from build123d import *

# Parameters (mm, degrees)
F0_W     = 906.4625
F0_H     = 547.6875
F1_DEPTH = 244.475
F2_W     = 21.43125
F2_H     = 490.5375
F3_DEPTH = 244.476
F4_R     = 25.4
F5_W     = 793.75
F5_H     = 455.6125
F6_DEPTH = 228.6
F7_R     = 25.4


with BuildPart() as f1:
    # F0 (on Top) → F1 (new body)
    with BuildSketch(Plane.XY):
        with Locations((15.469722, -72.404954)):
            Rectangle(F0_W, F0_H)
    extrude(amount=F1_DEPTH)

    # F2 (on face) → F3 (cut, through all)
    with BuildSketch(Plane.XY.offset(244.475)):
        with Locations((-427.045903, -43.829954)):
            Rectangle(F2_W, F2_H)
        with Locations((457.985347, -43.829954)):
            Rectangle(F2_W, F2_H)
    extrude(amount=-F3_DEPTH, mode=Mode.SUBTRACT)

    # F4
    f4_edges = [f1.edges().sort_by_distance(p)[0] for p in [
        (-437.761528, -346.248704, 122.2375),
        (468.700972, -346.248704, 122.2375),
    ]]
    fillet(f4_edges, radius=F4_R)

    # F5 (on face) → F6 (cut)
    with BuildSketch(Plane.XY.offset(244.475)):
        with Locations((15.469722, -61.292454)):
            Rectangle(F5_W, F5_H)
    extrude(amount=-F6_DEPTH, mode=Mode.SUBTRACT)

    # F7
    f7_edges = [f1.edges().sort_by_distance(p)[0] for p in [
        (412.344722, 166.513796, 130.175),
        (-381.405278, 166.513796, 130.175),
        (-381.405278, -289.098704, 130.175),
        (412.344722, -289.098704, 130.175),
    ]]
    fillet(f7_edges, radius=F7_R)


solid = f1.part
Here's how the part is built. I have some questions about the finished solid (model axes, mm). A direction names the side the tool comes from. Give positions to 0.01 mm unless a question says otherwise; leave off trailing zeros. Order: outer loops, then holes, each group sorted by start corner. A loop starts at its lowest first (then second) coordinate and runs counter-clockwise, first axis right, second up. Notation, with made-up numbers: (78.5, 7.25) -> (113.5, 7.25) arc R30 cw to (113.5, 36.25) -> close; hole circle Ø4 at (84.5, 35). An arc over 180 degrees is marked (long way). Use a Markdown table: item, result. Add a question column.
Item 1: For faces 1 (the face through (13, -294, 244.475)), 2 (the face through (-373.767, -281.856, 128.575)), 3 (the face through (447.27, -47, 124)), which set-ups out of +Z, -Z, +X, -X, +Y, -Y let a thin tool reach every point of the face, with its end or its side?
Item 2: Imagine slicing it at B-B on y = -94.5. Please give me the cut outline in (x, z) (3 decimals).
Item 3: Imagine slicing it at A-A on x = -345. Please give me the cut outline in (y, z) (3 decimals).
Item 4: Imagine slicing it at C-C on z = 28. Please give me the cut outline in (x, y), plus the area to 3 significant figures.
Item 5: I need wall thicknesses on line 1 (Y direction, x = -330, z = 144.5); line 2 (X direction, y = -234, z = 31); line 3 (Z direction, x = 212, y = -5.5) (3 decimals). Which ranges of each line are inside material? Lowest first, please.
Item 6: If we mould it in two halves opening along X, with no side actions, what happens to faces 4 (the face through (461.06, -339.01, 123.95)), 5 (the face through (-427, -289.099, 124)), 6 (the face through (405.1, 158.88, 128.57))? For each: pulls with the +X half, pulls with the -X half, needs draft (parallel to the pull), parting line crosses it, or undercut.
Item 7: Will these pins go through, and if not, where does the flat tip stop? pin 1 (6.5 mm diameter, centred on x = -425, z = 166.5, fed in from +Y); pin 2 (4 mm diameter, centred on y = 106.5, z = 75, fed in from +X); pin 3 (6 mm diameter, centred on x = 320.5, y = -58.5, fed in from +Z) (3 decimals).
Data:
| question | item | result |
|---|---|---|
| 1 | face 1 | +Z, +X, -X, +Y, -Y |
| 1 | face 2 | +Z |
| 1 | face 3 | +Z, -Z, +X, +Y |
| 2 | outline | (-416.33, 0) -> (447.27, 0) -> (447.27, 244.475) -> (412.345, 244.475) -> (412.345, 15.875) -> (-381.405, 15.875) -> (-381.405, 244.475) -> (-416.33, 244.475) -> close |
| 3 | outline | (-346.249, 0) -> (201.439, 0) -> (201.439, 244.475) -> (166.514, 244.475) -> (166.514, 15.875) -> (-289.099, 15.875) -> (-289.099, 244.475) -> (-346.249, 244.475) -> close |
| 4 | outline | (-437.76, -320.85) arc R25.4 ccw to (-412.36, -346.25) -> (443.3, -346.25) arc R25.4 ccw to (468.7, -320.85) -> (468.7, -289.1) -> (447.27, -289.1) -> (447.27, 201.44) -> (-416.33, 201.44) -> (-416.33, -289.1) -> (-437.76, -289.1) -> close; hole (-381.41, -263.7) arc R25.4 ccw to (-356.01, -289.1) -> (386.94, -289.1) arc R25.4 ccw to (412.34, -263.7) -> (412.34, 141.11) arc R25.4 ccw to (386.94, 166.51) -> (-356.01, 166.51) arc R25.4 ccw to (-381.41, 141.11) -> close |
| 4 | area | 114,000 mm² |
| 5 | line 1 | y = -346.25 to -289.1, 166.51 to 201.44 |
| 5 | line 2 | x = -416.33 to -381.41, 412.34 to 447.27 |
| 5 | line 3 | z = 0 to 15.875 |
| 6 | face 4 | pulls with the +X half |
| 6 | face 5 | needs draft |
| 6 | face 6 | undercut |
| 7 | pin 1 | stops at y = -289.1 |
| 7 | pin 2 | stops at x = 447.27 |
| 7 | pin 3 | stops at z = 15.875 |
